Input: part model. Units: mm. Frame: model coordinates. A direction names the side the tool comes from. Coordinates: 2 decimals unless noted, no trailing zeros. Loops run counter-clockwise (first coordinate to the right, second up) from the corner with the lowest first, then second, coordinate; pieces in that order, holes last.
Item 1: Reachability of faces 4 (the flat face through (2, -48, 115)), 5 (the flat face through (178.954, -47.779, 104.636)), 6 (the flat face through (-2, -25, -115)), 7 (the flat face through (-173, -49, 2)), 8 (the cylindrical face through (183.73, -47.78, -122.69)) from +Z, -Z, +X, -X, +Y, -Y: full face, straight path, thin tool, end or side. Return the list, or none.
Item 2: Section C-C on y = -12.5. Return loops of the section in (x, z).
Item 3: Pull-direction query (X, two-part tool) for faces 1 (the flat face through (44, 3, 2)), 2 (the flat face through (79, 0, 2)), 3 (the flat face through (-175, -48, 1)); classes: released by +X, released by -X, zero draft, split by the parting line, or undercut.
Item 4: Section A-A on x = -62. Return loops of the section in (y, z).
Item 5: Contact query for flat-ended pins moving along their axis: P1, Ø8, axis at x = -20.5, y = -58.5, coming from the -Z side; P2, Ø2.5, axis at x = -21, y = 1, coming from the +Z side; P3, Ø1.5, axis at y = -67.5, z = -44.5, coming from the +X side. Output: stop coordinate, or through.
Item 6: Section D-D on x = -125. Return loops of the section in (y, z), and give its area (3 significant figures).
Item 7: Section B-B on x = 134. Return loops of the section in (y, z).
Item 8: Ray query, line 1 along X through (y, z) = (0.5, 65); line 2 along X through (y, z) = (-17.5, -90); line 3 along Z through (x, y) = (47, 2). Return the intervals inside material, ascending.
Autodesk Inventor part; units mm, degrees
ref_plane "YZ Plane" through (0, 0, 0) normal (1, 0, 0) x (0, 1, 0)
ref_plane "XZ Plane" through (0, 0, 0) normal (0, 1, 0) x (-1, 0, 0)
ref_plane "XY Plane" through (0, 0, 0) normal (0, 0, 1) x (1, 0, 0)
sketch "Sketch1" plane through (0, 0, 0) normal (0, 1, 0) x (-1, 0, 0)
  line L0 (175, -115) -> (-175, -115)
  line L1 (-175, -115) -> (-175, 115)
  line L2 (-175, 115) -> (175, 115)
  line L3 (175, 115) -> (175, -115)
  line L4 (0, -115) -> (0, 115) construction
  line L5 (175, 0) -> (-175, 0) construction
  point P0 (0, 0)
  point P1 (0, 0)
  dimension "d0" = 350
  dimension "d1" = 230
extrude "Extrusion1" add sketch "Sketch1" along normal blind 3
sketch "Sketch6" plane through (0, 3, 0) normal (0, 1, 0) x (1, 0, 0)
  line L0 (175, 115) -> (-175, 115) construction
  line L1 (0, 115) -> (0, -115) construction
  line L2 (175, -115) -> (-175, -115) construction
  line L3 (-175, 115) -> (-175, -115) construction
  line L4 (-175, 0) -> (175, 0) construction
  line L5 (175, -115) -> (175, 115) construction
  circle A0 centre (-179, 119) radius 6
  line L6 (-175, 115) -> (-179, 115) construction
  line L7 (-179, 115) -> (-179, 119) construction
  line L8 (-179, 119) -> (-175, 119) construction
  line L9 (-175, 119) -> (-175, 115) construction
  line L10 (-155, 115) -> (-175.4528, 123.8392)
  line L11 (-175, 95) -> (-183.0203, 114.5461)
  line L12 (-175, 95) -> (-175, 115)
  line L13 (-155, 115) -> (-175, 115)
  circle A1 centre (-179, -119) radius 6
  line L14 (-155, -115) -> (-175.4528, -123.8392)
  line L15 (-175, -95) -> (-183.0203, -114.5461)
  line L16 (-175, -95) -> (-175, -115)
  line L17 (-155, -115) -> (-175, -115)
  circle A2 centre (179, 119) radius 6
  line L18 (155, 115) -> (175.4528, 123.8392)
  line L19 (175, 95) -> (183.0203, 114.5461)
  line L20 (175, 95) -> (175, 115)
  line L21 (155, 115) -> (175, 115)
  line L22 (175, -95) -> (183.0203, -114.5461)
  circle A3 centre (179, -119) radius 6
  line L23 (155, -115) -> (175.4528, -123.8392)
  line L24 (155, -115) -> (175, -115)
  line L25 (175, -95) -> (175, -115)
  circle A4 centre (179, -119) radius 2.75
  circle A5 centre (179, 119) radius 2.75
  circle A6 centre (-179, -119) radius 2.75
  circle A7 centre (-179, 119) radius 2.75
  point P0 (0, 0)
  dimension "d22" = 12
  dimension "d23" = 4
  dimension "d24" = 4
  dimension "d25" = 20
  dimension "d26" = 20
  dimension "d30" = 5.5
extrude "Extrusion6" add sketch "Sketch6" against normal blind 103 contours A0 L13 L12 | A0 L10 L13 | A0 L12 L11 | A1 L16 L17 | L15 L16 A1 | A1 L17 L14 | A2 L20 L21 | A2 L21 L18 | L19 L20 A2 | L22 A3 L25 | A3 L24 L25 | A3 L23 L24 | A4 | A5 | A6 | A7 picked at (-175.087, 116.3056) picked at (-175.087, -116.3056) picked at (175.0917, 116.2969) picked at (175.0917, -116.2969)
sketch "Sketch9" plane through (0, 0, 0) normal (0, -1, 0) x (1, 0, 0)
  line L0 (-175, -95) -> (-175, -115)
  line L1 (175, 115) -> (175, 95)
  line L2 (-175, -115) -> (175, -115)
  line L3 (175, -115) -> (175, 115)
  line L4 (175, 115) -> (-175, 115)
  line L5 (-175, 115) -> (-175, -115)
  line L6 (-173, -113) -> (173, -113)
  line L7 (173, -113) -> (173, 113)
  line L8 (173, 113) -> (-173, 113)
  line L9 (-173, 113) -> (-173, -113)
  line L10 (0, -115) -> (0, 115) construction
  line L11 (-155, 115) -> (155, 115) construction
  point P0 (0, 0)
  dimension "d31" = 2
  dimension "d32" = 2
  dimension "d33" = 2
  dimension "d34" = 2
extrude "Extrusion7" add sketch "Sketch9" along normal blind 100
sketch "Sketch10" plane through (155, 3, -115) normal (0, 0, -1) x (-1, 0, 0)
  line L0 (0, -103) -> (310, -103)
  line L1 (17, -103) -> (267, -103)
  line L2 (267, -103) -> (267, -48)
  line L3 (267, -48) -> (17, -48)
  line L4 (17, -48) -> (17, -103)
  line L5 (0, 0) -> (0, -103)
  line L6 (310, 0) -> (0, 0) construction
  line L7 (155, 0) -> (155, -103) construction
  line L8 (267, -48) -> (187, -48)
  line L9 (187, -48) -> (187, -23)
  line L10 (187, -23) -> (267, -23)
  line L11 (267, -23) -> (267, -48)
  point P0 (155, -3)
  point P1 (-18, -103)
  dimension "d38" = 55
  dimension "d39" = 35
  dimension "d40" = 250
  dimension "d41" = 25
  dimension "d42" = 80
extrude "Extrusion8" cut sketch "Sketch10" against normal up to next
sketch "Sketch11" plane through (0, 3, 0) normal (0, 1, 0) x (1, 0, 0)
  line L0 (-138, 90) -> (42, 90)
  line L1 (42, 90) -> (42, -60)
  line L2 (42, -60) -> (-138, -60)
  line L3 (-138, -60) -> (-138, 90)
  line L4 (-173, -113) -> (-173, 113)
  line L5 (-173, 113) -> (173, 113)
  point P0 (0, 0)
  dimension "d45" = 180
  dimension "d46" = 150
  dimension "d47" = 35
  dimension "d48" = 173
extrude "Extrusion9" cut sketch "Sketch11" against normal up to next
sketch "Sketch13" plane through (0, -100, 0) normal (0, -1, 0) x (1, 0, 0)
  arc A0 (-183.0203, -114.5461) -> (-175.4528, -123.8392) centre (-179, -119) ccw
  line L0 (-175, 95) -> (-175, -95) construction
  line L1 (-175, 0) -> (175, 0) construction
  line L2 (175, 95) -> (175, -95) construction
  line L3 (155, -115) -> (-155, -115) construction
  line L4 (0, -115) -> (0, 115) construction
  line L5 (-155, 115) -> (155, 115) construction
  circle A1 centre (-179, 119) radius 2.75
  circle A2 centre (179, 119) radius 2.75
  circle A3 centre (-179, -119) radius 2.75
  circle A4 centre (179, -119) radius 2.75
  point P0 (0, 0)
  dimension "d51" = 5.5
extrude "Extrusion10" cut sketch "Sketch13" against normal blind 7
sketch "Sketch14" plane through (0, 3, 0) normal (0, 1, 0) x (1, 0, 0)
  line L0 (-138, 90) -> (42, 90) construction
  line L1 (-138, -60) -> (-138, 90) construction
  line L2 (42, -60) -> (-138, -60) construction
  line L3 (42, 90) -> (42, -60) construction
  line L4 (-143, 95) -> (47, 95) construction
  line L5 (47, 95) -> (47, -65) construction
  line L6 (47, -65) -> (-143, -65) construction
  line L7 (-143, -65) -> (-143, 95) construction
  circle A0 centre (-143, 95) radius 3
  circle A1 centre (-143, 95) radius 1.75
  line L8 (-48, 95) -> (-48, -65) construction
  line L9 (-143, 15) -> (47, 15) construction
  circle A2 centre (47, 95) radius 3
  circle A3 centre (47, 95) radius 1.75
  circle A4 centre (-143, -65) radius 3
  circle A5 centre (-143, -65) radius 1.75
  circle A6 centre (47, -65) radius 3
  circle A7 centre (47, -65) radius 1.75
  point P0 (0, 0)
  dimension "d54" = 5
  dimension "d55" = 5
  dimension "d56" = 5
  dimension "d57" = 5
  dimension "d58" = 6
  dimension "d59" = 3.5
extrude "Extrusion11" cut sketch "Sketch14" against normal up to next contours A1 | A3 | A5 | A7
sketch "Sketch15" plane through (0, 3, 0) normal (0, 1, 0) x (1, 0, 0)
  circle A0 centre (47, 95) radius 1.75
  circle A1 centre (47, 95) radius 3.25
  line L0 (-138, 90) -> (42, 90) construction
  line L1 (42, 90) -> (42, -60) construction
  line L2 (42, -60) -> (-138, -60) construction
  line L3 (-138, -60) -> (-138, 90) construction
  line L4 (42, -60) -> (42, 90) construction
  line L5 (42, 15) -> (-138, 15) construction
  line L6 (-138, 90) -> (-138, -60) construction
  line L7 (42, 90) -> (-138, 90) construction
  line L8 (-48, 90) -> (-48, -60) construction
  circle A2 centre (47, -65) radius 3.25
  circle A3 centre (-143, 95) radius 3.25
  circle A4 centre (-143, -65) radius 3.25
  circle A5 centre (47, -65) radius 1.75
  circle A6 centre (-143, -65) radius 1.75
  circle A7 centre (-143, 95) radius 1.75
  point P0 (0, 0)
  dimension "d62" = 6.5
extrude "Extrusion12" add sketch "Sketch15" against normal blind 4
properties part number "vna_cover"
Results found:
1. face 4: +Z, +Y, -Y
1. face 5: +X, +Y, -Y
1. face 6: -Z, +Y, -Y
1. face 7: -Y
1. face 8: +Y, -Y
2. outline: (-183.02, -114.55) arc R6 ccw to (-175.45, -123.84) - (-155, -115) - (155, -115) - (175.45, -123.84) arc R6 ccw to (183.02, -114.55) - (175, -95) - (175, 95) - (183.02, 114.55) arc R6 ccw to (175.45, 123.84) - (155, 115) - (-155, 115) - (-175.45, 123.84) arc R6 ccw to (-183.02, 114.55) - (-175, 95) - (-175, -95) - close; hole (-173, -113) - (173, -113) - (173, 113) - (-173, 113) - close
3. face 1: zero draft
3. face 2: undercut
3. face 3: released by -X
4. outline: (-100, 113) - (0, 113) - (0, 60) - (3, 60) - (3, 115) - (-100, 115) - close; (-20, -115) - (3, -115) - (3, -90) - (0, -90) - (0, -113) - (-20, -113) - close
5. P1: stops at z = 113
5. P2: stops at z = 115
5. P3: stops at x = 175
6. outline: (-100, -115) - (3, -115) - (3, -90) - (0, -90) - (0, -113) - (-100, -113) - close; (-100, 113) - (0, 113) - (0, 60) - (3, 60) - (3, 115) - (-100, 115) - close
6. area: 640 mm2
7. outline: (-100, 113) - (0, 113) - (0, -113) - (-45, -113) - (-45, -115) - (3, -115) - (3, 115) - (-100, 115) - close
8. line 1: x = -175 to -144.75, -141.25 to 45.25, 48.75 to 175
8. line 2: x = -175 to -173, 173 to 175
8. line 3: z = -115 to -96.75, -93.25 to 63.25, 66.75 to 115
